```python
from build123d import *

# Parameters (mm, degrees)
F1_DEPTH       = 615
F3_DEPTH       = 60
F5_D           = 9
F5_CSINK_D     = 20
F5_CSINK_ANGLE = 90


with BuildPart() as f1:
    # F0 (on Right) → F1 (new body)
    with BuildSketch(Plane.YZ):
        Polygon((0, 5), (0, 0), (60, 0), (60, 60), (55, 60), (55, 5), align=None)
    extrude(amount=F1_DEPTH)

    # F2 (on face) → F3 (cut, through all)
    with BuildSketch(Plane(origin=(0, 0, 0), x_dir=(1, 0, 0), z_dir=(0, 0, -1))):
        Polygon((0, 0), (0, -60), (60, 0), align=None)
        Polygon((555, 0), (615, -60), (615, 0), align=None)
    extrude(amount=-F3_DEPTH, mode=Mode.SUBTRACT)

    # F5 (through all)
    with Locations(Plane.XZ.offset(-55)):
        with Locations((35, 46), (20, 19), (580, 46), (595, 19)):
            CounterSinkHole(F5_D / 2, F5_CSINK_D / 2, counter_sink_angle=F5_CSINK_ANGLE)


solid = f1.part
```
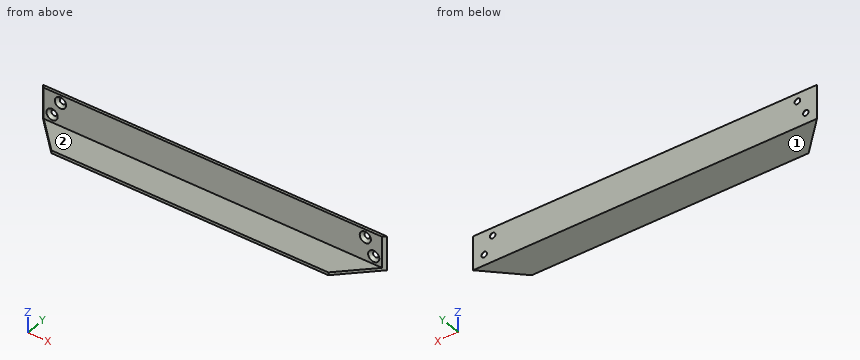
The listing builds one solid part. Answer for the finished solid, in the listing's coordinates (mm). Face numbers are marked on the shaded views. A direction names the side the tool comes from. Round coordinates to 2 decimals unless told otherwise and drop trailing zeros. Write each loop counter-clockwise with the first axis right and the second up, starting at its lowest first coordinate (ties: lowest second). Pieces come first, ordered by that corner, then holes. Notation, with made-up numbers: (35, -13) -> (60, -13) arc R20 cw to (60, 1) -> close; hole circle Ø10 at (-2, 46). An arc over 180 degrees is marked (long way). Use CSV: the item, a comma, the result in double quotes. Start each with the question number.
(1) Section D-D on y = 14 is taken. Give the vertices of the cut face in (x, z), then the cut area to 4 significant figures.
(2) Section B-B on x = 595 is taken. Give the vertices of the cut face in (y, z).
(3) Which of the six approach directions +Z, -Z, +X, -X, +Y, -Y give full straight-line access (tool end or side, diameter ignored) to the marked faces 1 and 2?
(4) Section C-C on x = 83 is taken. Give the vertices of the cut face in (y, z).
(5) This flat-tipped pin is pushed along its axis until it touches: pin 1 (16.5 mm diameter, centred on x = 202, y = 28, fed in from +Z). Where does it stop, or does it pass through?
(6) Section A-A on z = 19 is taken. Give the vertices of the cut face in (x, y).
(7) Consider L1, parallel to Y at x = 110.5, z = 41; L2, parallel to Z at x = 477, y = 22; L3, parallel to X at y = 57.5, z = 16. Determine where each line is inside the solid, lowest interval first. Write a range as from..to.
A:
1,outline,"(46, 0) -> (569, 0) -> (569, 5) -> (46, 5) -> close"
1,area,"2,615 mm²"
2,outline,"(40, 0) -> (60, 0) -> (60, 14) -> (55, 9) -> (55, 5) -> (40, 5) -> close; (55, 29) -> (60, 24) -> (60, 60) -> (55, 60) -> close"
3,face 1,"-Z, +X, -X, +Y, -Y"
3,face 2,"+Z, +X, -X, -Y"
4,outline,"(0, 0) -> (60, 0) -> (60, 60) -> (55, 60) -> (55, 5) -> (0, 5) -> close"
5,pin 1,"stops at z = 5"
6,outline,"(0, 60) -> (5, 55) -> (10, 55) -> (15, 60) -> close; (25, 60) -> (30, 55) -> (585, 55) -> (590, 60) -> close; (600, 60) -> (605, 55) -> (610, 55) -> (615, 60) -> close"
7,L1,"y = 55..60"
7,L2,"z = 0..5"
7,L3,"x = 2.5..13.13, 26.87..588.13, 601.87..612.5"
